```python
from build123d import *

# Parameters (mm, degrees)
SKETCH_1_W          = 85
SKETCH_1_H          = 65
SKETCH_1_R          = 4
EXTRUDE_1_DEPTH     = 6
SKETCH_2_R          = 2.5
CUT_EXTRUDE_1_DEPTH = 108.172757733


with BuildPart() as part:
    # Эскиз1 → Вытянуть1 (new body)
    with BuildSketch(Plane(origin=(0, 0, 0), x_dir=(1, 0, 0), z_dir=(0, 1, 0))):
        with Locations((42.5, -32.5)):
            Rectangle(SKETCH_1_W, SKETCH_1_H)
        with Locations(Location((42.5, -32.5, 0), (0, 0, 270))):
            Circle(SKETCH_1_R, mode=Mode.SUBTRACT)
    extrude(amount=EXTRUDE_1_DEPTH)

    # Эскиз2 → Вырез-Вытянуть1 (cut, through all)
    with BuildSketch(Plane(origin=(0, 6, 0), x_dir=(1, 0, 0), z_dir=(0, 1, 0))):
        with Locations(Location((77, -57, 0), (0, 0, 270))):
            Circle(SKETCH_2_R)
    extrude(amount=-CUT_EXTRUDE_1_DEPTH, mode=Mode.SUBTRACT)


solid = part.part
```
Input: part model. Units: mm. Frame: model coordinates. Round coordinates to 2 decimals unless told otherwise and drop trailing zeros. Write each loop counter-clockwise with the first axis right and the second up, starting at its lowest first coordinate (ties: lowest second). Pieces come first, ordered by that corner, then holes. Notation, with made-up numbers: (69.25, 48) -> (91.25, 48) arc R6 ccw to (91.25, 53) -> close; hole circle Ø10 at (37.5, -20.75). An arc over 180 degrees is marked (long way). Answer as CSV lines item,"result".
1. Section B-B (z = 57). Return the cut outline in (x, y).
Geometry says:
outline,"(0, 0) -> (74.5, 0) -> (74.5, 6) -> (0, 6) -> close; (79.5, 0) -> (85, 0) -> (85, 6) -> (79.5, 6) -> close"
2. Contact query for a flat-ended pin moving along its axis: P1, Ø13, axis at x = 42.5, z = 32.5, coming from the +Y side. Output: stop coordinate, or through.
Geometry says:
P1,"stops at y = 6"
3. Section A-A (x = 42.5). Return the cut outline in (y, z), plus the area to 3 significant figures.
Geometry says:
outline,"(0, 0) -> (6, 0) -> (6, 28.5) -> (0, 28.5) -> close; (0, 36.5) -> (6, 36.5) -> (6, 65) -> (0, 65) -> close"
area,"342 mm^2"
4. Mould query, pull axis X, two halves, no side actions, for faces 1 (the flat face through (42, 6, 25)), 2 (the flat face through (0, 3, 33)), 3 (the cylindrical face through (76.04, 3.04, 59.31)). Classes: +X half, -X half, draft (parallel to the pull), parting line (faces both ways), or undercut.
Geometry says:
face 1,"draft"
face 2,"-X half"
face 3,"undercut"
5. Ray query, L1, parallel to X at y = 4.2, z = 32.5; L2, parallel to Z at x = 41, y = 1.4; L3, parallel to X at y = 1.9, z = 35. Return the intervals inside material, ascending. Write a range as [from, to].
Geometry says:
L1,"x = [0, 38.5], [46.5, 85]"
L2,"z = [0, 28.79], [36.21, 65]"
L3,"x = [0, 39.38], [45.62, 85]"
